Job drawing, mm, ordinate dimensions from the low corner. One solid piece. Give positions to 0.01 mm unless a question says otherwise; leave off trailing zeros. Loops run counter-clockwise (first coordinate to the right, second up) from the corner with the lowest first, then second, coordinate; pieces in that order, holes last. Notation, with made-up numbers: M -28,-20 L 1,-20 A18 cw 1,-14 Z; hole C 84.25,-34.75 d11. An arc over 180 degrees is marked long. Answer as CSV lines item,"result".
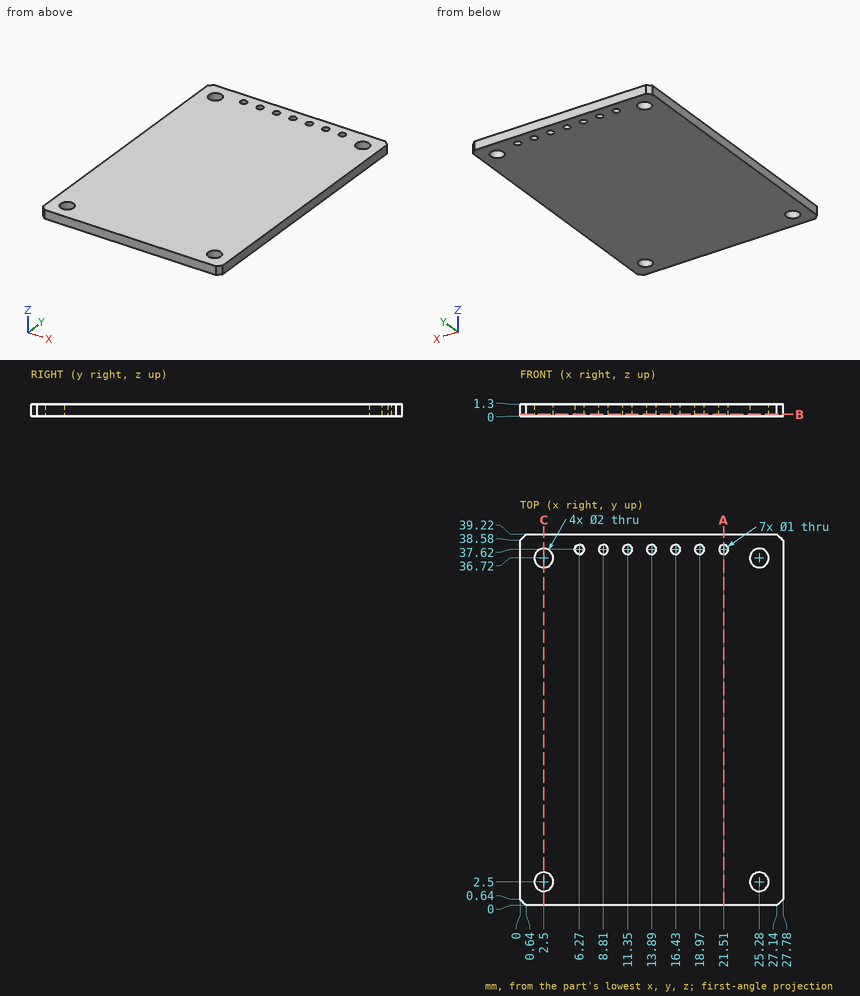
1) Drill centre lines: line 1 (Y direction, x = 25.25, z = 1.1); line 2 (X direction, y = 36.72, z = 1); line 3 (Y direction, x = 8.81, z = 0.65). Where is each one in solid material? Low to high. Write a range as from..to.
Answer below:
line 1,"y = 0..1.5, 3.5..35.72, 37.72..39.22"
line 2,"x = 0..1.5, 3.5..24.28, 26.28..27.78"
line 3,"y = 0..37.12, 38.12..39.22"
2) Band-saw the part on C-C on x = 2.5. Give the cut face in (y, z).
Answer below:
outline,"M 0,0 L 1.5,0 L 1.5,1.3 L 0,1.3 Z; M 3.5,0 L 35.72,0 L 35.72,1.3 L 3.5,1.3 Z; M 37.72,0 L 39.22,0 L 39.22,1.3 L 37.72,1.3 Z"
3) Band-saw the part on A-A on x = 21.51. Give the cut face in (y, z), and give its area (3 significant figures).
Answer below:
outline,"M 0,0 L 37.12,0 L 37.12,1.3 L 0,1.3 Z; M 38.12,0 L 39.22,0 L 39.22,1.3 L 38.12,1.3 Z"
area,"49.7 mm^2"
4) Band-saw the part on B-B on z = 0.2. Give the number of separate pieces and of enclosed holes in the cut face, and give its area (3 significant figures).
Answer below:
separate pieces,"1"
enclosed holes,"11"
area,"1,070 mm^2"
5) Flat gauge pins, fed straight in: pin 1 (2.5 mm diameter, centred on x = 25.28, y = 2.5, fed in from +Z); pin 2 (1.8 mm diameter, centred on x = 2.5, y = 36.72, fed in from +Z). Where does each tip first touch, or does it go through?
Answer below:
pin 1,"stops at z = 1.3"
pin 2,"passes through"
